Source: CAD feature listing. Evaluate the final solid. Frame: model axes, mm. A direction names the side the tool comes from. Round coordinates to 2 decimals unless told otherwise and drop trailing zeros. Order: outer loops, then holes, each group sorted by start corner. A loop starts at its lowest first (then second) coordinate and runs counter-clockwise, first axis right, second up. Notation, with made-up numbers: (-7, 77.25) -> (13, 77.25) arc R17 cw to (13, 104.25) -> close; hole circle Ø9 at (84, 52.25). An arc over 180 degrees is marked (long way). Write item = value, one per line. Start each with the question number.
(1) Contact query for flat-ended pins moving along their axis: pin 1 Ø11 at (x, y) = (-7.5, -1) entering from +Z; pin 2 Ø4 at (x, z) = (1.5, 2.5) entering from +Y; pin 3 Ø0.5 at (y, z) = (2.5, 6) entering from -X. Output: stop coordinate, or through.
(2) Cut plane B-B on z = 5. Return the cut outline in (x, y), then the cut area to 3 significant figures.
(3) Reachability of faces 4 (the face through (0, -2.3, 9)), 5 (the face through (0, 0, 0)), 6 (the face through (0, 13, 1)) from +Z, -Z, +X, -X, +Y, -Y: full face, straight path, thin tool, end or side. Return the list, or none.
(4) Ray query, line 1 (X direction, y = 8, z = 7); line 2 (X direction, y = 6.5, z = 12); line 3 (Y direction, x = 10, z = 4.5). Return the intervals inside material, ascending.
(5) Cut plane C-C on z = 11. Return the cut outline in (x, y), then the cut area to 3 significant figures.
(6) Cut plane A-A on z = 8. Return the cut outline in (x, y), then the cut area to 3 significant figures.
(7) Draft query along Y for faces 1 (the face through (6, -19, 15)), 2 (the face through (-4.351, -19.596, 5.728)), 3 (the face through (0.5, 13.4, 0.5)). Return one class per face: released by +Y, released by -Y, zero draft, split by the parting line, or undercut.
(8) Cut plane D-D on z = 14.25. Return the cut outline in (x, y) (3 decimals), then the cut area to 3 significant figures.
from build123d import *

# Parameters (mm, degrees)
F0_R     = 21
F1_DEPTH = 15
F2_DEPTH = 1.5
F3_DEPTH = 1
F4_DEPTH = 9
F5_SIZE2 = 1.49999
F5_SIZE  = 14.99999


# Not quite as in the source:
# - a fillet or chamfer that OpenCascade refuses, or shapes differently, is made with other operations: its cross-section is extruded or revolved along the edge and cut away or added
# - a fillet or chamfer is up to 0.001 mm smaller than in the source, because OpenCascade refuses the exact size


with BuildPart() as f1:
    # F0 (on Top) → F1 (new body)
    with BuildSketch(Plane.XY):
        Circle(F0_R)
        with BuildLine():
            ThreePointArc((0.5, 18.4932420089), (13.2570735836, 12.9034879006), (18.5, 0))
            ThreePointArc((18.5, 0), (-12.9034879006, -13.2570735836), (-0.5, 18.4932420089))
            ThreePointArc((-0.5, 18.4932420089), (0, 18.5), (0.5, 18.4932420089))
        make_face(mode=Mode.SUBTRACT)
    extrude(amount=F1_DEPTH)

    # F0 (on Top) → F2 (join)
    with BuildSketch(Plane.XY):
        with BuildLine():
            ThreePointArc((-0.5, 18.4932420089), (-12.9034879006, -13.2570735836), (18.5, 0))
            ThreePointArc((18.5, 0), (13.2570735836, 12.9034879006), (0.5, 18.4932420089))
            Line((0.5, 18.4932420089), (0.5, 8.4932420089))
            ThreePointArc((0.5, 8.4932420089), (0, 7.9932420089), (-0.5, 8.4932420089))
            Line((-0.5, 8.4932420089), (-0.5, 18.4932420089))
        make_face()
        with BuildLine():
            ThreePointArc((0.25, 2.9895651858), (2.2079402166, 2.0310096012), (3, 0))
            ThreePointArc((3, 0), (2.9276371182, -0.6549358016), (2.7140393972, -1.2782762419))
            ThreePointArc((2.7140393972, -1.2782762419), (2.5980762114, -1.5), (2.4640393972, -1.7112889438))
            ThreePointArc((2.4640393972, -1.7112889438), (0, -3), (-2.4640393972, -1.7112889438))
            ThreePointArc((-2.4640393972, -1.7112889438), (-2.5980762114, -1.5), (-2.7140393972, -1.2782762419))
            ThreePointArc((-2.7140393972, -1.2782762419), (-2.5980762114, 1.5), (-0.25, 2.9895651858))
            ThreePointArc((-0.25, 2.9895651858), (0, 3), (0.25, 2.9895651858))
        make_face(mode=Mode.SUBTRACT)
        with BuildLine():
            ThreePointArc((2, 0), (1.5, 1.3228756555), (0.25, 1.9843134833))
            ThreePointArc((0.25, 1.9843134833), (0, 2), (-0.25, 1.9843134833))
            ThreePointArc((-0.25, 1.9843134833), (-1.7320508076, 1), (-1.8434658856, -0.7756503907))
            ThreePointArc((-1.8434658856, -0.7756503907), (-1.7320508076, -1), (-1.5934658856, -1.2086630926))
            ThreePointArc((-1.5934658856, -1.2086630926), (0, -2), (1.5934658856, -1.2086630926))
            ThreePointArc((1.5934658856, -1.2086630926), (1.7320508076, -1), (1.8434658856, -0.7756503907))
            ThreePointArc((1.8434658856, -0.7756503907), (1.9604759334, -0.3956439237), (2, 0))
        make_face()
        with BuildLine():
            Line((0.5, 8.4932420089), (0.5, 18.4932420089))
            Line((0.5, 18.4932420089), (-0.5, 18.4932420089))
            Line((-0.5, 18.4932420089), (-0.5, 8.4932420089))
            ThreePointArc((-0.5, 8.4932420089), (0, 8.9932420089), (0.5, 8.4932420089))
        make_face()
        with BuildLine():
            Line((-0.25, 1.9843134833), (-0.25, 2.9895651858))
            ThreePointArc((-0.25, 2.9895651858), (-2.5980762114, 1.5), (-2.7140393972, -1.2782762419))
            Line((-2.7140393972, -1.2782762419), (-1.8434658856, -0.7756503907))
            ThreePointArc((-1.8434658856, -0.7756503907), (-1.7320508076, 1), (-0.25, 1.9843134833))
        make_face()
        with BuildLine():
            ThreePointArc((-2.4640393972, -1.7112889438), (0, -3), (2.4640393972, -1.7112889438))
            Line((2.4640393972, -1.7112889438), (1.5934658856, -1.2086630926))
            ThreePointArc((1.5934658856, -1.2086630926), (0, -2), (-1.5934658856, -1.2086630926))
            Line((-1.5934658856, -1.2086630926), (-2.4640393972, -1.7112889438))
        make_face()
        with BuildLine():
            ThreePointArc((2.7140393972, -1.2782762419), (2.9276371182, -0.6549358016), (3, 0))
            ThreePointArc((3, 0), (2.2079402166, 2.0310096012), (0.25, 2.9895651858))
            Line((0.25, 2.9895651858), (0.25, 1.9843134833))
            ThreePointArc((0.25, 1.9843134833), (1.5, 1.3228756555), (2, 0))
            ThreePointArc((2, 0), (1.9604759334, -0.3956439237), (1.8434658856, -0.7756503907))
            Line((1.8434658856, -0.7756503907), (2.7140393972, -1.2782762419))
        make_face()
        with BuildLine():
            Line((0.25, 1.9843134833), (0.25, 2.9895651858))
            ThreePointArc((0.25, 2.9895651858), (0, 3), (-0.25, 2.9895651858))
            Line((-0.25, 2.9895651858), (-0.25, 1.9843134833))
            ThreePointArc((-0.25, 1.9843134833), (0, 2), (0.25, 1.9843134833))
        make_face()
        with BuildLine():
            ThreePointArc((2.4640393972, -1.7112889438), (2.5980762114, -1.5), (2.7140393972, -1.2782762419))
            Line((2.7140393972, -1.2782762419), (1.8434658856, -0.7756503907))
            ThreePointArc((1.8434658856, -0.7756503907), (1.7320508076, -1), (1.5934658856, -1.2086630926))
            Line((1.5934658856, -1.2086630926), (2.4640393972, -1.7112889438))
        make_face()
        with BuildLine():
            Line((-1.8434658856, -0.7756503907), (-2.7140393972, -1.2782762419))
            ThreePointArc((-2.7140393972, -1.2782762419), (-2.5980762114, -1.5), (-2.4640393972, -1.7112889438))
            Line((-2.4640393972, -1.7112889438), (-1.5934658856, -1.2086630926))
            ThreePointArc((-1.5934658856, -1.2086630926), (-1.7320508076, -1), (-1.8434658856, -0.7756503907))
        make_face()
        with BuildLine():
            ThreePointArc((-0.5, 8.4932420089), (0, 7.9932420089), (0.5, 8.4932420089))
            Line((0.5, 8.4932420089), (-0.5, 8.4932420089))
        make_face()
        with BuildLine():
            Line((-0.5, 8.4932420089), (0.5, 8.4932420089))
            ThreePointArc((0.5, 8.4932420089), (0, 8.9932420089), (-0.5, 8.4932420089))
        make_face()
        with BuildLine():
            Line((-0.5, 18.4932420089), (0.5, 18.4932420089))
            ThreePointArc((0.5, 18.4932420089), (0, 18.5), (-0.5, 18.4932420089))
        make_face()
    extrude(amount=F2_DEPTH)

    # F0 (on Top) → F3 (cut)
    with BuildSketch(Plane.XY):
        with BuildLine():
            ThreePointArc((-0.5, 8.4932420089), (0, 7.9932420089), (0.5, 8.4932420089))
            Line((0.5, 8.4932420089), (-0.5, 8.4932420089))
        make_face()
        with BuildLine():
            Line((-0.5, 8.4932420089), (0.5, 8.4932420089))
            ThreePointArc((0.5, 8.4932420089), (0, 8.9932420089), (-0.5, 8.4932420089))
        make_face()
        with BuildLine():
            Line((-0.5, 18.4932420089), (0.5, 18.4932420089))
            ThreePointArc((0.5, 18.4932420089), (0, 18.5), (-0.5, 18.4932420089))
        make_face()
        with BuildLine():
            Line((0.5, 8.4932420089), (0.5, 18.4932420089))
            Line((0.5, 18.4932420089), (-0.5, 18.4932420089))
            Line((-0.5, 18.4932420089), (-0.5, 8.4932420089))
            ThreePointArc((-0.5, 8.4932420089), (0, 8.9932420089), (0.5, 8.4932420089))
        make_face()
    extrude(amount=F3_DEPTH, mode=Mode.SUBTRACT)

    # F0 (on Top) → F4 (join)
    with BuildSketch(Plane.XY):
        with BuildLine():
            Line((-0.25, 1.9843134833), (-0.25, 2.9895651858))
            ThreePointArc((-0.25, 2.9895651858), (-2.5980762114, 1.5), (-2.7140393972, -1.2782762419))
            Line((-2.7140393972, -1.2782762419), (-1.8434658856, -0.7756503907))
            ThreePointArc((-1.8434658856, -0.7756503907), (-1.7320508076, 1), (-0.25, 1.9843134833))
        make_face()
        with BuildLine():
            ThreePointArc((2.7140393972, -1.2782762419), (2.9276371182, -0.6549358016), (3, 0))
            ThreePointArc((3, 0), (2.2079402166, 2.0310096012), (0.25, 2.9895651858))
            Line((0.25, 2.9895651858), (0.25, 1.9843134833))
            ThreePointArc((0.25, 1.9843134833), (1.5, 1.3228756555), (2, 0))
            ThreePointArc((2, 0), (1.9604759334, -0.3956439237), (1.8434658856, -0.7756503907))
            Line((1.8434658856, -0.7756503907), (2.7140393972, -1.2782762419))
        make_face()
        with BuildLine():
            ThreePointArc((-2.4640393972, -1.7112889438), (0, -3), (2.4640393972, -1.7112889438))
            Line((2.4640393972, -1.7112889438), (1.5934658856, -1.2086630926))
            ThreePointArc((1.5934658856, -1.2086630926), (0, -2), (-1.5934658856, -1.2086630926))
            Line((-1.5934658856, -1.2086630926), (-2.4640393972, -1.7112889438))
        make_face()
    extrude(amount=F4_DEPTH)

    # F5 (size 15 and 1.5 in the source; OpenCascade refuses exactly that, so slightly less here)
    f5_edges = [f1.edges().sort_by_distance(p)[0] for p in [
        (-21, 0, 0),
    ]]
    f5_side = f1.faces().sort_by_distance((-21, 0, 7.5))[0]
    chamfer(f5_edges, length=F5_SIZE, length2=F5_SIZE2, reference=f5_side)

    # F6: chamfer of 14 x 1 on 1 edges, made by hand


with BuildPart() as f6_tool2:
    # F6_s3 → F6_t4 (revolve)
    with BuildSketch(Plane(origin=(0, 0, 0), x_dir=(0, 0, 1), z_dir=(0.9996347032, 0.027027027, 0))):
        Polygon((15, -19.5), (1, -18.5), (15, -18.5), align=None)
    revolve(axis=Axis((0, 0, 15), (0, 0, 1)))

    split(bisect_by=Plane.XY.offset(1.5), keep=Keep.TOP)


with BuildPart() as f1_1:
    add(f1.part)

    # F6_t1: cut F6_tool2
    add(f6_tool2.part, mode=Mode.SUBTRACT)


solid = f1_1.part
Evaluation:
q1.pin_1 = 9
q1.pin_2 = 19.92
q1.pin_3 = -19.98
q2.outline = circle Ø40 at (0, 0); (-2.71, -1.28) -> (-1.84, -0.78) arc R2 cw to (-0.25, 1.98) -> (-0.25, 2.99) arc R3 ccw to start; (-2.46, -1.71) arc R3 ccw to (2.46, -1.71) -> (1.59, -1.21) arc R2 cw to (-1.59, -1.21) -> close; (0.25, 1.98) arc R2 cw to (1.84, -0.78) -> (2.71, -1.28) arc R3 ccw to (0.25, 2.99) -> close; hole circle Ø37.57 at (0, 0)
q2.area = 162 mm^2
q3.face_4 = +Z
q3.face_5 = -Z, +X, -X, +Y, -Y
q3.face_6 = -Z
q4.line_1 = -18.55 to -17.15, 17.15 to 18.55
q4.line_2 = -19.65 to -18.16, 18.16 to 19.65
q4.line_3 = -17.26 to -15.86, 15.86 to 17.26
q5.outline = circle Ø41.2 at (0, 0); hole circle Ø38.43 at (0, 0)
q5.area = 173 mm^2
q6.outline = circle Ø40.6 at (0, 0); (-2.71, -1.28) -> (-1.84, -0.78) arc R2 cw to (-0.25, 1.98) -> (-0.25, 2.99) arc R3 ccw to start; (-2.46, -1.71) arc R3 ccw to (2.46, -1.71) -> (1.59, -1.21) arc R2 cw to (-1.59, -1.21) -> close; (0.25, 1.98) arc R2 cw to (1.84, -0.78) -> (2.71, -1.28) arc R3 ccw to (0.25, 2.99) -> close; hole circle Ø38 at (0, 0)
q6.area = 175 mm^2
q7.face_1 = zero draft
q7.face_2 = split by the parting line
q7.face_3 = undercut
q8.outline = circle Ø41.85 at (0, 0); hole circle Ø38.893 at (0, 0)
q8.area = 188 mm^2
